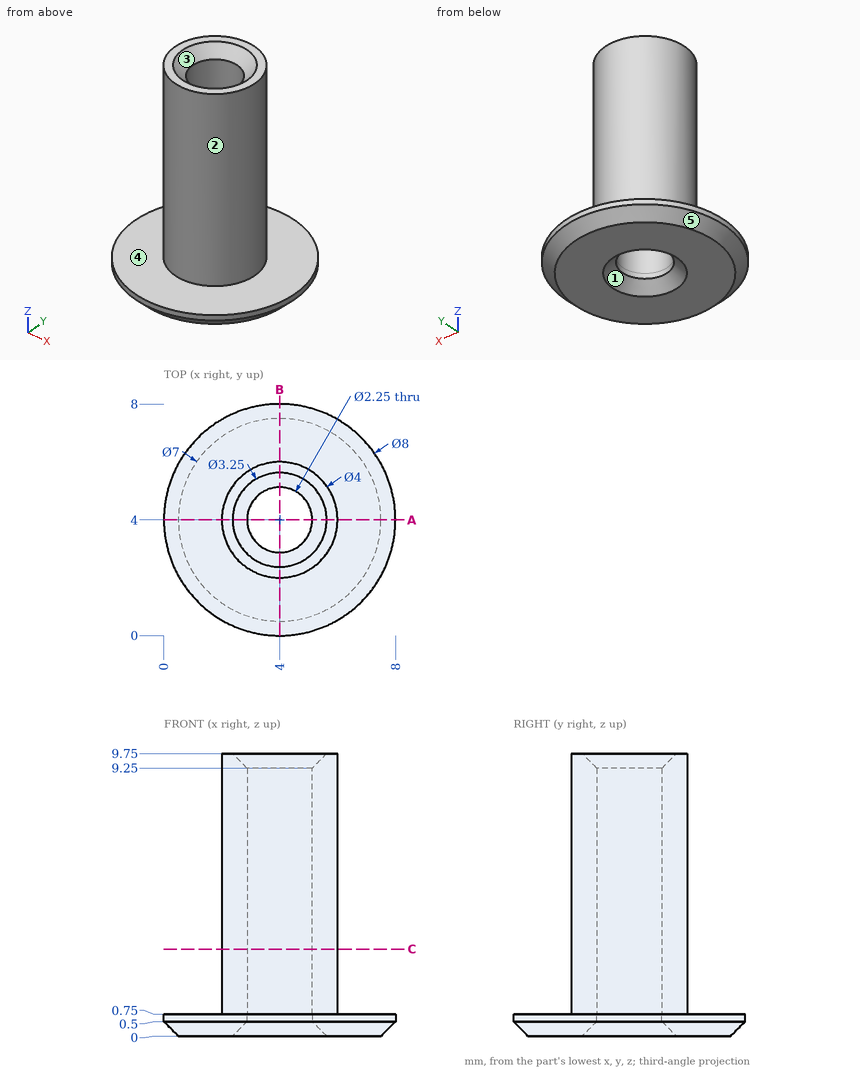
Could you check a few things on this drawing? It's one solid part, dimensions in mm from its lowest x, y, z. A direction names the side the tool comes from. Give positions to 0.01 mm unless a question says otherwise; leave off trailing zeros. Order: outer loops, then holes, each group sorted by start corner. A loop starts at its lowest first (then second) coordinate and runs counter-clockwise, first axis right, second up. Notation, with made-up numbers: M -40,77.25 L -21,77.25 A8 cw -21,82.25 Z; hole C -24,4 d3. An arc over 180 degrees is marked long. Use one line per item in the form item = value.
Item 1: Will these pins go through, and if not, where does the flat tip stop? pin 1 Ø1.8 at (x, y) = (4, 4) entering from -Z; pin 2 Ø3 at (x, y) = (4, 4) entering from +Z (3 decimals); pin 3 Ø2 at (y, z) = (4.5, 4.5) entering from -X; pin 4 Ø2 at (y, z) = (4, 7) entering from +X.
Values follow:
pin_1 = through
pin_2 = 9.625
pin_3 = 2
pin_4 = 6
Item 2: If I drill on line 1 along Y through (x, z) = (4, 5.5) (3 decimals); line 2 along Y through (x, z) = (4, 0.65) (3 decimals); line 3 along Z through (x, y) = (4, 1.25), over which ranges is the centre line in solid material (lowest first)? Write a range as [from, to].
Values follow:
line_1 = [2, 2.875], [5.125, 6]
line_2 = [0, 2.875], [5.125, 8]
line_3 = [0, 0.75]
Item 3: If we section it at C-C, the plane z = 3: Write out the boundary of the cut face in (x, y) (3 decimals).
Values follow:
outline = C 4,4 d4; hole C 4,4 d2.25
Item 4: For the marked faces 1 and 2, which set-ups out of +Z, -Z, +X, -X, +Y, -Y let a thin tool reach every point of the face, with its end or its side?
Values follow:
face_1 = -Z
face_2 = +Z
Item 5: Thinking about a two-plate mould opening in Y: for the marked faces 3, 4 and 5, which applies, pulls with the +Y half, pulls with the -Y half, needs draft (parallel to the pull), parting line crosses it, or undercut?
Values follow:
face_3 = undercut
face_4 = needs draft
face_5 = parting line crosses it
Item 6: If we section it at A-A, the plane y = 4: Write out the boundary of the cut face in (x, z) (3 decimals).
Values follow:
outline = M 0,0.5 L 0.5,0 L 2.375,0 L 2.875,0.5 L 2.875,9.25 L 2.375,9.75 L 2,9.75 L 2,0.75 L 0,0.75 Z; M 5.125,0.5 L 5.625,0 L 7.5,0 L 8,0.5 L 8,0.75 L 6,0.75 L 6,9.75 L 5.625,9.75 L 5.125,9.25 Z
